from build123d import *

# Parameters (mm, degrees)
SKETCH1_R             = 2.2479
EXTRUDE1_DEPTH        = 9.017
SKETCH2_R             = 19.05
EXTRUDE2_DEPTH        = 1.524
SKETCH3_R             = 3.175
EXTRUDE3_DEPTH        = 23.8
EXTRUDE5_DEPTH        = 34
CUT_EXTRUDE2_START    = -34
CUT_EXTRUDE2_DEPTH    = 34
EXTRUDE7_DEPTH        = 11.5
CUT_EXTRUDE3_START    = -48
CUT_EXTRUDE3_DEPTH    = 48
EXTRUDE8_DEPTH        = 5
CHANFRO1_SIZE         = 0.5
ESBO_O1_R             = 1
CORTE_EXTRUS_O1_DEPTH = 2


with BuildPart() as part:
    # Sketch1 → Extrude1 (new body)
    with BuildSketch(Plane.XY):
        with BuildLine():
            Line((-4.572, 0), (-51.816, 0))
            ThreePointArc((-51.816, 0), (-55.048892204, 1.339107796), (-56.388, 4.572))
            Line((-56.388, 4.572), (-56.388, 51.816))
            ThreePointArc((-56.388, 51.816), (-55.048892204, 55.048892204), (-51.816, 56.388))
            Line((-51.816, 56.388), (-4.572, 56.388))
            ThreePointArc((-4.572, 56.388), (-1.339107796, 55.048892204), (0, 51.816))
            Line((0, 51.816), (0, 4.572))
            ThreePointArc((0, 4.572), (-1.339107796, 1.339107796), (-4.572, 0))
        make_face()
        with Locations((-4.572, 51.816)):
            Circle(SKETCH1_R, mode=Mode.SUBTRACT)
        with Locations((-4.572, 4.572)):
            Circle(SKETCH1_R, mode=Mode.SUBTRACT)
        with Locations((-51.816, 4.572)):
            Circle(SKETCH1_R, mode=Mode.SUBTRACT)
        with Locations((-51.816, 51.816)):
            Circle(SKETCH1_R, mode=Mode.SUBTRACT)
    extrude(amount=-EXTRUDE1_DEPTH)

    # Sketch2 → Extrude2 (add)
    with BuildSketch(Plane.XY):
        with Locations(Location((-28.194, 28.194, 0), (0, 0, 180))):
            Circle(SKETCH2_R)
    extrude(amount=EXTRUDE2_DEPTH)

    # Sketch3 → Extrude3 (add)
    with BuildSketch(Plane.XY.offset(1.524)):
        with Locations((-28.194, 28.194)):
            Circle(SKETCH3_R)
    extrude(amount=EXTRUDE3_DEPTH)

    # Sketch5 → Extrude5 (add)
    with BuildSketch(Plane(origin=(0, 0, -9.017), x_dir=(-1, 0, 0), z_dir=(0, 0, -1))):
        with BuildLine():
            Line((4.572, 0.0254), (51.816, 0.0254))
            ThreePointArc((51.816, 0.0254), (55.030931691, 1.357068309), (56.3626, 4.572))
            Line((56.3626, 4.572), (56.3626, 51.816))
            ThreePointArc((56.3626, 51.816), (55.030931691, 55.030931691), (51.816, 56.3626))
            Line((51.816, 56.3626), (4.572, 56.3626))
            ThreePointArc((4.572, 56.3626), (1.357068309, 55.030931691), (0.0254, 51.816))
            Line((0.0254, 51.816), (0.0254, 4.572))
            ThreePointArc((0.0254, 4.572), (1.357068309, 1.357068309), (4.572, 0.0254))
        make_face()
    extrude(amount=EXTRUDE5_DEPTH)

    # Sketch7 → Cut-Extrude2 (cut)
    with BuildSketch(Plane(origin=(0, 0, -43.017), x_dir=(-1, 0, 0), z_dir=(0, 0, -1)).offset(CUT_EXTRUDE2_START)):
        with BuildLine():
            Line((2.098933629, 46.697411693), (6.801120561, 47.526534117))
            ThreePointArc((6.801120561, 47.526534117), (8.156105414, 48.231894586), (8.861465883, 49.586879439))
            Line((8.861465883, 49.586879439), (9.690588307, 54.289066371))
            ThreePointArc((9.690588307, 54.289066371), (10.559319471, 55.793752886), (12.192, 56.388))
            Line((12.192, 56.388), (4.572, 56.388))
            ThreePointArc((4.572, 56.388), (1.339107796, 55.048892204), (0, 51.816))
            Line((0, 51.816), (0, 44.196))
            ThreePointArc((0, 44.196), (0.594247114, 45.828680529), (2.098933629, 46.697411693))
        make_face()
        with BuildLine():
            Line((56.388, 51.816), (56.388, 44.196))
            ThreePointArc((56.388, 44.196), (55.793752886, 45.828680529), (54.289066371, 46.697411693))
            Line((54.289066371, 46.697411693), (49.586879439, 47.526534117))
            ThreePointArc((49.586879439, 47.526534117), (48.231894586, 48.231894586), (47.526534117, 49.586879439))
            Line((47.526534117, 49.586879439), (46.697411693, 54.289066371))
            ThreePointArc((46.697411693, 54.289066371), (45.828680529, 55.793752886), (44.196, 56.388))
            Line((44.196, 56.388), (51.816, 56.388))
            ThreePointArc((51.816, 56.388), (55.048892204, 55.048892204), (56.388, 51.816))
        make_face()
        with BuildLine():
            Line((54.289066371, 9.690588307), (49.586879439, 8.861465883))
            ThreePointArc((49.586879439, 8.861465883), (48.231894586, 8.156105414), (47.526534117, 6.801120561))
            Line((47.526534117, 6.801120561), (46.697411693, 2.098933629))
            ThreePointArc((46.697411693, 2.098933629), (45.828680529, 0.594247114), (44.196, 0))
            Line((44.196, 0), (51.816, 0))
            ThreePointArc((51.816, 0), (55.048892204, 1.339107796), (56.388, 4.572))
            Line((56.388, 4.572), (56.388, 12.192))
            ThreePointArc((56.388, 12.192), (55.793752886, 10.559319471), (54.289066371, 9.690588307))
        make_face()
        with BuildLine():
            Line((0, 4.572), (0, 12.192))
            ThreePointArc((0, 12.192), (0.594247114, 10.559319471), (2.098933629, 9.690588307))
            Line((2.098933629, 9.690588307), (6.801120561, 8.861465883))
            ThreePointArc((6.801120561, 8.861465883), (8.156105414, 8.156105414), (8.861465883, 6.801120561))
            Line((8.861465883, 6.801120561), (9.690588307, 2.098933629))
            ThreePointArc((9.690588307, 2.098933629), (10.559319471, 0.594247114), (12.192, 0))
            Line((12.192, 0), (4.572, 0))
            ThreePointArc((4.572, 0), (1.339107796, 1.339107796), (0, 4.572))
        make_face()
    extrude(amount=CUT_EXTRUDE2_DEPTH, mode=Mode.SUBTRACT)

    # Sketch6 → Extrude7 (add)
    with BuildSketch(Plane(origin=(0, 0, -43.017), x_dir=(-1, 0, 0), z_dir=(0, 0, -1))):
        with BuildLine():
            Line((0, 51.816), (0, 4.572))
            ThreePointArc((0, 4.572), (1.339107796, 1.339107796), (4.572, 0))
            Line((4.572, 0), (51.816, 0))
            ThreePointArc((51.816, 0), (55.048892204, 1.339107796), (56.388, 4.572))
            Line((56.388, 4.572), (56.388, 51.816))
            ThreePointArc((56.388, 51.816), (55.048892204, 55.048892204), (51.816, 56.388))
            Line((51.816, 56.388), (4.572, 56.388))
            ThreePointArc((4.572, 56.388), (1.339107796, 55.048892204), (0, 51.816))
        make_face()
    extrude(amount=EXTRUDE7_DEPTH)

    # Sketch8 → Cut-Extrude3 (cut)
    with BuildSketch(Plane(origin=(0, 0, -54.517), x_dir=(-1, 0, 0), z_dir=(0, 0, -1)).offset(CUT_EXTRUDE3_START)):
        with BuildLine():
            Line((2.098933629, 46.722811693), (6.779527926, 47.548126753))
            ThreePointArc((6.779527926, 47.548126753), (8.134512779, 48.253487221), (8.839873247, 49.608472074))
            Line((8.839873247, 49.608472074), (9.665188307, 54.289066371))
            ThreePointArc((9.665188307, 54.289066371), (10.533919471, 55.793752886), (12.1666, 56.388))
            Line((12.1666, 56.388), (4.572, 56.388))
            ThreePointArc((4.572, 56.388), (1.339107796, 55.048892204), (0, 51.816))
            Line((0, 51.816), (0, 44.2214))
            ThreePointArc((0, 44.2214), (0.594247114, 45.854080529), (2.098933629, 46.722811693))
        make_face()
        with BuildLine():
            Line((56.388, 51.816), (56.388, 44.2214))
            ThreePointArc((56.388, 44.2214), (55.793752886, 45.854080529), (54.289066371, 46.722811693))
            Line((54.289066371, 46.722811693), (49.608472074, 47.548126753))
            ThreePointArc((49.608472074, 47.548126753), (48.253487221, 48.253487221), (47.548126753, 49.608472074))
            Line((47.548126753, 49.608472074), (46.722811693, 54.289066371))
            ThreePointArc((46.722811693, 54.289066371), (45.854080529, 55.793752886), (44.2214, 56.388))
            Line((44.2214, 56.388), (51.816, 56.388))
            ThreePointArc((51.816, 56.388), (55.048892204, 55.048892204), (56.388, 51.816))
        make_face()
        with BuildLine():
            Line((54.289066371, 9.665188307), (49.608472074, 8.839873247))
            ThreePointArc((49.608472074, 8.839873247), (48.253487221, 8.134512779), (47.548126753, 6.779527926))
            Line((47.548126753, 6.779527926), (46.722811693, 2.098933629))
            ThreePointArc((46.722811693, 2.098933629), (45.854080529, 0.594247114), (44.2214, 0))
            Line((44.2214, 0), (51.816, 0))
            ThreePointArc((51.816, 0), (55.048892204, 1.339107796), (56.388, 4.572))
            Line((56.388, 4.572), (56.388, 12.1666))
            ThreePointArc((56.388, 12.1666), (55.793752886, 10.533919471), (54.289066371, 9.665188307))
        make_face()
        with BuildLine():
            Line((0, 4.572), (0, 12.1666))
            ThreePointArc((0, 12.1666), (0.594247114, 10.533919471), (2.098933629, 9.665188307))
            Line((2.098933629, 9.665188307), (6.779527926, 8.839873247))
            ThreePointArc((6.779527926, 8.839873247), (8.134512779, 8.134512779), (8.839873247, 6.779527926))
            Line((8.839873247, 6.779527926), (9.665188307, 2.098933629))
            ThreePointArc((9.665188307, 2.098933629), (10.533919471, 0.594247114), (12.1666, 0))
            Line((12.1666, 0), (4.572, 0))
            ThreePointArc((4.572, 0), (1.339107796, 1.339107796), (0, 4.572))
        make_face()
    extrude(amount=CUT_EXTRUDE3_DEPTH, mode=Mode.SUBTRACT)

    # Sketch9 → Extrude8 (add)
    with BuildSketch(Plane.XZ):
        Polygon((-38.444, -54.517), (-17.944, -54.517), (-17.944, -43.017), (-18.944, -43.017), (-18.944, -50.517), (-37.444, -50.517), (-37.444, -43.017), (-38.444, -43.017), align=None)
    extrude(amount=EXTRUDE8_DEPTH)

    # Chanfro1
    chanfro1_edges = [part.edges().sort_by_distance(p)[0] for p in [
        (-31.369, 28.194, 25.324),
    ]]
    chamfer(chanfro1_edges, length=CHANFRO1_SIZE)

    # Esboço1 → Corte-extrusão1 (cut)
    with BuildSketch(Plane.XY.offset(25.324)):
        with Locations((-28.194, 28.194)):
            Circle(ESBO_O1_R)
    extrude(amount=-CORTE_EXTRUS_O1_DEPTH, mode=Mode.SUBTRACT)

    # Esboço2 → Corte-Revolução1 (revolve, cut)
    with BuildSketch(Plane(origin=(0, 28.194, 0), x_dir=(-1, 0, 0), z_dir=(0, 1, 0))):
        Polygon((11.194, 1.524), (13.194, -0.476), (15.194, -0.476), (15.194, 1.524), align=None)
    revolve(axis=Axis((-28.194, 28.194, 25.324), (0, 0, -1)), mode=Mode.SUBTRACT)


solid = part.part
Verification items for the finished model (mm, model axes). A direction names the side the tool comes from. Give positions to 0.01 mm unless a question says otherwise; leave off trailing zeros. Loops run counter-clockwise (first coordinate to the right, second up) from the corner with the lowest first, then second, coordinate; pieces in that order, holes last.
1. Cross-section at A-A on y = 5.5. Count the separate pieces of the cut face and the enclosed holes in it, and give its area (3 significant figures).
Derived:
separate pieces: 3
enclosed holes: 0
area: 2,150 mm2
2. Material ranges on probe 1 along Y at (x, z) = (-37.5, -1); probe 2 along X at (y, z) = (37, -40); probe 3 along Z at (x, y) = (-33, 30.5), recorded low to high.
Derived:
probe 1: y = 0 to 56.39
probe 2: x = -56.36 to -0.03
probe 3: z = -54.52 to 1.52
3. Release check for a two-part mould opening along X. For faces 1 (the flat face through (-28, 27, 25.324)), 2 (the flat face through (-37.444, -2, -47)), 3 (the flat face through (-4.41, 47.13, -7.75)) record: +X half, -X half, draft (parallel to the pull), parting line (faces both ways), or undercut.
Derived:
face 1: draft
face 2: undercut
face 3: +X half
4. Cross-section at C-C on z = 18. Record the cut outline in (x, y) (3 decimals), and give its area (3 significant figures).
Derived:
outline: circle Ø6.35 at (-28.194, 28.194)
area: 31.7 mm2
5. Tool access check on faces 4 (the cylindrical face through (-27.27, 27.81, 24.34)), 5 (the cylindrical face through (-55.81, 10.553, -48.686)), 6 (the flat face through (-15, 0, -49)). Record the directions out of +Z, -Z, +X, -X, +Y, -Y that give a thin tool (end or side, any length) a straight path to the whole face; none if there is none.
Derived:
face 4: +Z
face 5: -Z, -X, -Y
face 6: +Z, -Z, +X, -Y
6. Cross-section at B-B on z = -27. Record the cut outline in (x, y).
Derived:
outline: (-56.36, 11.83) arc R2.54 ccw to (-54.29, 9.69) - (-49.59, 8.86) arc R2.54 cw to (-47.53, 6.8) - (-46.7, 2.1) arc R2.54 ccw to (-44.55, 0.03) - (-11.83, 0.03) arc R2.54 ccw to (-9.69, 2.1) - (-8.86, 6.8) arc R2.54 cw to (-6.8, 8.86) - (-2.1, 9.69) arc R2.54 ccw to (-0.03, 11.83) - (-0.03, 44.55) arc R2.54 ccw to (-2.1, 46.7) - (-6.8, 47.53) arc R2.54 cw to (-8.86, 49.59) - (-9.69, 54.29) arc R2.54 ccw to (-11.83, 56.36) - (-44.55, 56.36) arc R2.54 ccw to (-46.7, 54.29) - (-47.53, 49.59) arc R2.54 cw to (-49.59, 47.53) - (-54.29, 46.7) arc R2.54 ccw to (-56.36, 44.55) - close
7. Go/stop test with flat-tipped pins: P1, Ø3, axis at x = -10.5, y = 9.5, coming from the +Z side; P2, Ø6, axis at y = 49, z = 1, coming from the -X side; P3, Ø10, axis at x = -29, z = -26, coming from the +Y side; P4, Ø6, axis at y = 47.5, z = -29.5, coming from the +X side. Record where each tip stops, or that it passes through.
Derived:
P1: stops at z = 0
P2: stops at x = -56.39
P3: stops at y = 56.36
P4: stops at x = -0.03
